Autodesk Inventor part; units mm, degrees
ref_plane "Work Plane1" through (0, 0, 55) normal (0, 0, 1) x (1, 0, 0)
ref_plane "YZ Plane" through (0, 0, 0) normal (1, 0, 0) x (0, 1, 0)
ref_plane "XZ Plane" through (0, 0, 0) normal (0, 1, 0) x (-1, 0, 0)
sketch "Sketch1" plane through (0, 0, 0) normal (0, 0, 1) x (1, 0, 0)
  circle A0 centre (0, 0) radius 5
  circle A1 centre (0, 0) radius 9.5
  circle A2 centre (0, 0) radius 8.5
  dimension "d" = 10
  dimension "D" = 19
  dimension "d23" = 17
extrude "Extrusion1" add sketch "Sketch1" along normal blind 49 contours A1 | A2
sketch "Sketch2" plane through (0, 0, 49) normal (0, 0, 1) x (1, 0, 0)
  circle A0 centre (0, 0) radius 9.5
  line L0 (-15, -15) -> (15, -15)
  line L1 (15, -15) -> (15, 15)
  line L2 (15, 15) -> (-15, 15)
  line L3 (-15, 15) -> (-15, -15)
  line L4 (-15, -15) -> (15, 15) construction
  line L5 (15, -15) -> (-15, 15) construction
  circle A1 centre (0, 0) radius 14.5 construction
  circle A2 centre (10.253, 10.253) radius 2.25
  circle A3 centre (10.253, 10.253) radius 3.75
  line L6 (-5.4596, 0) -> (5.4596, 0) construction
  line L7 (0, -5.5798) -> (0, 5.5798) construction
  circle A4 centre (10.253, -10.253) radius 2.25
  circle A5 centre (10.253, -10.253) radius 3.75
  circle A6 centre (-10.253, 10.253) radius 2.25
  circle A7 centre (-10.253, 10.253) radius 3.75
  circle A8 centre (-10.253, -10.253) radius 3.75
  circle A9 centre (-10.253, -10.253) radius 2.25
  circle A10 centre (0, 0) radius 5
  point P0 (15, 0)
  point P1 (0, 15)
  point P2 (0, 0)
  point P3 (0, 0)
  dimension "DP" = 29
  dimension "k" = 30
  dimension "d27" = 30
  dimension "X" = 4.5
  dimension "Y" = 7.5
ref_plane "Work Plane1" through (0, 0, 55) normal (0, 0, 1) x (1, 0, 0)
extrude "Extrusion6" cut sketch "Sketch1" along normal blind 1 contours A2
extrude "Extrusion7" add sketch "Sketch2" along normal blind 6 contours L3 L2 L1 L0
chamfer "Chamfer1" distance 2 angle 45 4 edges at (-15, -15, 52) (15, -15, 52) (15, 15, 52) (-15, 15, 52)
extrude "Extrusion8" add sketch "Sketch2" along normal blind 1.9 contours A3 | A5 | A7 | A8
extrude "Extrusion9" add sketch "Sketch2" along normal blind 5 contours A0
chamfer "Chamfer2" distance 0.2 angle 45 16 edges at (0, -15, 55) (-15, 0, 55) (0, 15, 55) (15, 0, 55) (14, -14, 55) (-14, -14, 55) (-14, 14, 55) (14, 14, 55) (-14, -14, 49) (0, -15, 49) (-15, 0, 49) (14, -14, 49) (15, 0, 49) (14, 14, 49) (0, 15, 49) (-14, 14, 49)
equation "\"d27\" = k"
equation "\"d36\" = t - z"
equation "\"z\" = 4.1"
properties part number "RolamentoLinear10d"
CAD build for the part. Positions are in the model's coordinates, mm. A direction names the side the tool comes from. Coordinates: 2 decimals unless noted, no trailing zeros. Order: outer loops, then holes, each group sorted by start corner. A loop starts at its lowest first (then second) coordinate and runs counter-clockwise, first axis right, second up. Notation, with made-up numbers: (37.25, 7.5) - (94.25, 7.5) arc R22 cw to (94.25, 19.5) - close; hole circle Ø8 at (33.25, 51.25). An arc over 180 degrees is marked (long way). Use a Markdown table: item, result. Add a question column.
(1) Saw through at D-D (y = 11.5). Give the cut face in (x, z), then the cut area to 3 significant figures.
(2) Saw through at C-C (z = 43). Give the cut face in (x, y).
(3) Flat gauge pins, fed straight in: pin 1 (2 mm diameter, centred on x = -10.5, y = -10, fed in from +Z); pin 2 (1.5 mm diameter, centred on y = 8, z = 7, fed in from +X); pin 3 (8.5 mm diameter, centred on x = 10.253, y = 10.253, fed in from -Z); pin 4 (1.5 mm diameter, centred on x = 7, z = 9.5, fed in from +Y). Where does each tip first touch, or does it go through?
(4) Drill centre lines: line 1 along Z through (x, y) = (-13.5, 7); line 2 along Z through (x, y) = (5, 5); line 3 along Y through (x, z) = (0, 54.7). Where is each one in solid material? Low to high. Write a range as [from, to].
(5) Which spindle directions (+Z, -Z, +X, -X, +Y, -Y) get a long thin tool onto all of the face, cutting with end or side? Do faces 1 (the face through (4, -4, 1)), 2 (the face through (-11.066, 13.914, 52.921)), 3 (the face through (-2.2, -8.4, 0)). Say none if no direction does.
(6) Saw through at A-A (x = 0). Give the cut face in (y, z), then the cut area to 3 significant figures.
(7) Pull direction Y, two halves, no side cores. Call faces 4 (the face through (4.38, 8.43, 24.16)), 5 (the face through (-1.08, 4.88, 27.13)), 6 (the face through (14, 14, 52)): +Y half, -Y half, draft (parallel to the pull), parting line (faces both ways), or undercut.
Solved:
| question | item | result |
|---|---|---|
| 1 | outline | (-15, 49.2) - (-14.8, 49) - (-12.13, 49) - (-12.13, 50.9) - (-13.79, 50.9) - (-13.79, 55) - (-14.8, 55) - (-15, 54.8) - close; (-8.38, 49) - (8.38, 49) - (8.38, 50.9) - (6.72, 50.9) - (6.72, 55) - (-6.72, 55) - (-6.72, 50.9) - (-8.38, 50.9) - close; (12.13, 49) - (14.8, 49) - (15, 49.2) - (15, 54.8) - (14.8, 55) - (13.79, 55) - (13.79, 50.9) - (12.13, 50.9) - close |
| 1 | area | 108 mm² |
| 2 | outline | circle Ø19 at (0, 0); hole circle Ø10 at (0, 0) |
| 3 | pin 1 | passes through |
| 3 | pin 2 | stops at x = 6.14 |
| 3 | pin 3 | stops at z = 49 |
| 3 | pin 4 | stops at y = 7.15 |
| 4 | line 1 | z = [49, 55] |
| 4 | line 2 | z = [1, 54] |
| 4 | line 3 | y = [-15, -9.5], [9.5, 15] |
| 5 | face 1 | -Z |
| 5 | face 2 | +Z |
| 5 | face 3 | -Z, +X, -X, +Y, -Y |
| 6 | outline | (-15, 49.2) - (-14.8, 49) - (-9.5, 49) - (-9.5, 0) - (-8.5, 0) - (-8.5, 1) - (-5, 1) - (-5, 54) - (-9.5, 54) - (-9.5, 55) - (-14.8, 55) - (-15, 54.8) - close; (5, 1) - (8.5, 1) - (8.5, 0) - (9.5, 0) - (9.5, 49) - (14.8, 49) - (15, 49.2) - (15, 54.8) - (14.8, 55) - (9.5, 55) - (9.5, 54) - (5, 54) - close |
| 6 | area | 545 mm² |
| 7 | face 4 | parting line |
| 7 | face 5 | undercut |
| 7 | face 6 | +Y half |
